from build123d import *

# Parameters (mm, degrees)
BOSS_EXTRUDE1_DEPTH = 20
SKETCH2_R           = 1.25
BOSS_EXTRUDE2_DEPTH = 6
SKETCH3_R           = 1.25
CUT_EXTRUDE1_DEPTH  = 6


with BuildPart() as part:
    # Sketch1 → Boss-Extrude1 (new body)
    with BuildSketch(Plane(origin=(0, 0, 0), x_dir=(1, 0, 0), z_dir=(0, 1, 0))):
        Polygon((-2.886751346, 0), (-1.443375673, -2.5), (1.443375673, -2.5), (2.886751346, 0), (1.443375673, 2.5), (-1.443375673, 2.5), align=None)
    extrude(amount=BOSS_EXTRUDE1_DEPTH)

    # Sketch2 → Boss-Extrude2 (add)
    with BuildSketch(Plane(origin=(0, 20, 0), x_dir=(1, 0, 0), z_dir=(0, 1, 0))):
        Circle(SKETCH2_R)
    extrude(amount=BOSS_EXTRUDE2_DEPTH)

    # Sketch3 → Cut-Extrude1 (cut)
    with BuildSketch(Plane.XZ):
        Circle(SKETCH3_R)
    extrude(amount=-CUT_EXTRUDE1_DEPTH, mode=Mode.SUBTRACT)


solid = part.part
Verification items for the finished model (mm, model axes). A direction names the side the tool comes from. Give positions to 0.01 mm unless a question says otherwise; leave off trailing zeros. Loops run counter-clockwise (first coordinate to the right, second up) from the corner with the lowest first, then second, coordinate; pieces in that order, holes last. Notation, with made-up numbers: (80, 60.25) - (126, 60.25) arc R18 cw to (126, 82.25) - close; hole circle Ø9 at (50.25, 80.5). An arc over 180 degrees is marked (long way). Write item = value, one per line. Start each with the question number.
Q1. Tool access check on faces 5 (the face through (-0.27, 22.96, 1.22)), 6 (the face through (-0.27, 2.96, -1.22)), 7 (the face through (0, 26, 0)). Record the directions out of +Z, -Z, +X, -X, +Y, -Y that give a thin tool (end or side, any length) a straight path to the whole face; none if there is none.
Q2. Cross-section at B-B, the plane z = 0.45. Enter the section's corners in (x, y), and give its area (3 significant figures).
Q3. Depth check by flat-ended pin: P1, Ø2, axis at x = 0, z = 0, coming from the -Y side. Enter the tip coordinate at first touch or a pass-through.
Q4. Cross-section at D-D, the plane y = 21.25. Enter the section's corners in (x, z).
Q5. Cross-section at C-C, the plane x = 0.3. Enter the section's corners in (y, z), and give its area (3 significant figures).
Q6. Thickness scan on line 1 (Z direction, x = 0, y = 4.4); line 2 (Y direction, x = -1.65, z = -0.15); line 3 (Y direction, x = 1, z = -0.2). Record the ranges inside material, lowest first.
Q7. Cross-section at A-A, the plane y = 14. Enter the section's corners in (x, z).
Q8. Mould release check, pull along Z, two halves, no side actions. Record for faces 1 (the face through (0, 6, 0)), 2 (the face through (1, 0, -1)), 3 (the face through (0, 10, -2.5)), 4 (the face through (-2.175, 9.86, 1.233)): released by +Z, released by -Z, zero draft, split by the parting line, or undercut.
Answer key:
q1.face_5 = +Y
q1.face_6 = -Y
q1.face_7 = +Z, -Z, +X, -X, +Y
q2.outline = (-2.63, 0) - (-1.17, 0) - (-1.17, 6) - (1.17, 6) - (1.17, 0) - (2.63, 0) - (2.63, 20) - (1.17, 20) - (1.17, 26) - (-1.17, 26) - (-1.17, 20) - (-2.63, 20) - close
q2.area = 105 mm^2
q3.P1 = 6
q4.outline = circle Ø2.5 at (0, 0)
q5.outline = (0, -2.5) - (20, -2.5) - (20, -1.21) - (26, -1.21) - (26, 1.21) - (20, 1.21) - (20, 2.5) - (0, 2.5) - (0, 1.21) - (6, 1.21) - (6, -1.21) - (0, -1.21) - close
q5.area = 100 mm^2
q6.line_1 = -2.5 to -1.25, 1.25 to 2.5
q6.line_2 = 0 to 20
q6.line_3 = 6 to 26
q7.outline = (-2.89, 0) - (-1.44, -2.5) - (1.44, -2.5) - (2.89, 0) - (1.44, 2.5) - (-1.44, 2.5) - close
q8.face_1 = undercut
q8.face_2 = zero draft
q8.face_3 = released by -Z
q8.face_4 = released by +Z
